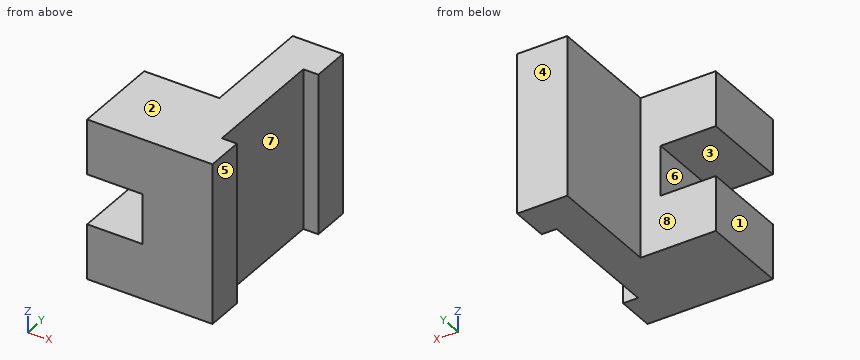
```python
from build123d import *

# Parameters (mm, degrees)
BOSS_EXTRUDE1_DEPTH = 64
SKETCH4_W           = 20
SKETCH4_H           = 35
CUT_EXTRUDE2_DEPTH  = 22


with BuildPart() as part:
    # Sketch2 → Boss-Extrude1 (new body)
    with BuildSketch(Plane.XY):
        Polygon((0, 0), (50, 0), (50, 15), (44, 15), (44, 65), (50, 65), (50, 80), (30, 80), (30, 35), (0, 35), align=None)
    extrude(amount=BOSS_EXTRUDE1_DEPTH)

    # Sketch4 → Cut-Extrude2 (cut)
    with BuildSketch(Plane.ZY):
        with Locations((32, 17.5)):
            Rectangle(SKETCH4_W, SKETCH4_H)
    extrude(amount=-CUT_EXTRUDE2_DEPTH, mode=Mode.SUBTRACT)


solid = part.part
```
Design review of the part built by this model. Coordinates are the model's own, in mm. Face numbers are marked on the shaded views. A direction names the side the tool comes from. Round coordinates to 2 decimals unless told otherwise and drop trailing zeros. Order: outer loops, then holes, each group sorted by start corner. A loop starts at its lowest first (then second) coordinate and runs counter-clockwise, first axis right, second up. Notation, with made-up numbers: (27.5, 78.5) - (82.5, 78.5) arc R16 cw to (82.5, 109.5) - close; hole circle Ø8 at (19.25, -1.75). An arc over 180 degrees is marked (long way). Return JSON: item names as keys, results as strings.
Q1. Wall thickness on L1, parallel to Y at x = 45, z = 29.5; L2, parallel to X at y = 69, z = 19.5; L3, parallel to X at y = 38.5, z = 46.5: over which ranges is each line inside the solid? List them lowest first. Write a range as [from, to].
Computed values:
{"L1": "y = [0, 15], [65, 80]", "L2": "x = [30, 50]", "L3": "x = [30, 44]"}
Q2. For pin 1 Ø15 at (y, z) = (32.5, 45.5) entering from +X; pin 2 Ø24 at (x, z) = (7.5, 29.5) entering from +Y; pin 3 Ø3 at (y, z) = (38, 35) entering from -X, all flat-tipped, find the tip position at first contact; note any pin that passes through.
Computed values:
{"pin 1": "stops at x = 44", "pin 2": "stops at y = 35", "pin 3": "stops at x = 30"}
Q3. Consider section D-D on y = 10.5. Write out the cut boundary in (x, z), plus the area to 3 significant figures.
Computed values:
{"outline": "(0, 0) - (50, 0) - (50, 64) - (0, 64) - (0, 42) - (22, 42) - (22, 22) - (0, 22) - close", "area": "2,760 mm2"}
Q4. Machinability: for the marked faces 4, 5, 6, 7 and 8, which of the approach directions +Z, -Z, +X, -X, +Y, -Y give a long, thin tool a straight path to every point of the face, cutting with its end or side? Answer none if there is none.
Computed values:
{"face 4": "+Z, -Z, +X, -X, +Y", "face 5": "+Z, -Z, +X, +Y, -Y", "face 6": "-X, +Y, -Y", "face 7": "+Z, -Z, +X", "face 8": "+Z, -Z, -X, +Y"}
Q5. The part is to be moulded in two halves that separate along Z. For the marked faces 1, 2 and 3, say which applies: pulls with the +Z half, pulls with the -Z half, needs draft (parallel to the pull), parting line crosses it, or undercut.
Computed values:
{"face 1": "needs draft", "face 2": "pulls with the +Z half", "face 3": "undercut"}
Q6. Consider section A-A on x = 19. Write out the cut boundary in (y, z), plus the area to 3 significant figures.
Computed values:
{"outline": "(0, 0) - (35, 0) - (35, 22) - (0, 22) - close; (0, 42) - (35, 42) - (35, 64) - (0, 64) - close", "area": "1,540 mm2"}
Q7. Consider section B-B on y = 25. Write out the cut boundary in (x, z), plus the area to 3 significant figures.
Computed values:
{"outline": "(0, 0) - (44, 0) - (44, 64) - (0, 64) - (0, 42) - (22, 42) - (22, 22) - (0, 22) - close", "area": "2,380 mm2"}
Q8. Consider section C-C on z = 39.5. Write out the cut boundary in (x, y), plus the area to 3 significant figures.
Computed values:
{"outline": "(22, 0) - (50, 0) - (50, 15) - (44, 15) - (44, 65) - (50, 65) - (50, 80) - (30, 80) - (30, 35) - (22, 35) - close", "area": "1,580 mm2"}
